The figure shows three views and two pictorial views of one solid part (mm, origin at its lowest corner). Answer the questions. A direction names the side the tool comes from. Round coordinates to 2 decimals unless told otherwise and drop trailing zeros. Write each loop counter-clockwise with the first axis right and the second up, starting at its lowest first coordinate (ties: lowest second). Pieces come first, ordered by that corner, then holes. Notation, with made-up numbers: M 66,64 L 121,64 A19 cw 121,91 Z; hole C 29.5,3.25 d6. An arc over 180 degrees is marked long. One line per item, written item: value. Start each with the question number.
Q1. Find section D-D (x = 4). Write down the section's boundary in (y, z).
Q2. The mould has two halves that part along X. Classify the marked faces 1, 2 and 3: released by +X, released by -X, zero draft, split by the parting line, or undercut.
Q3. Consider probe 1 along Y at (x, z) = (7.5, 1.25); probe 2 along Y at (x, z) = (7.5, 4.55); probe 3 along Z at (x, y) = (10.75, 4.5). Determine where each line is inside the solid, lowest interval first.
Q4. Given pin 1 Ø1 at (y, z) = (10, 3) entering from +X; pin 2 Ø2 at (y, z) = (13, 2) entering from -X; pin 3 Ø1.5 at (x, z) = (11.5, 5.5) entering from -Y, each flat-ended and moving along its own axis, determine where each tip first touches the part or whether it passes through.
Q5. A tool of negligible diameter and unlimited length cuts with its end or side. For the marked faces 4 and 5, from which of +Z, -Z, +X, -X, +Y, -Y can it reach the whole face along a straight path? Write none if from no direction.
Q6. Find section A-A (y = 7.5). Write down the section's boundary in (x, z), and give its area (3 significant figures).
Q7. Find section C-C (z = 1). Write down the section's boundary in (x, y).
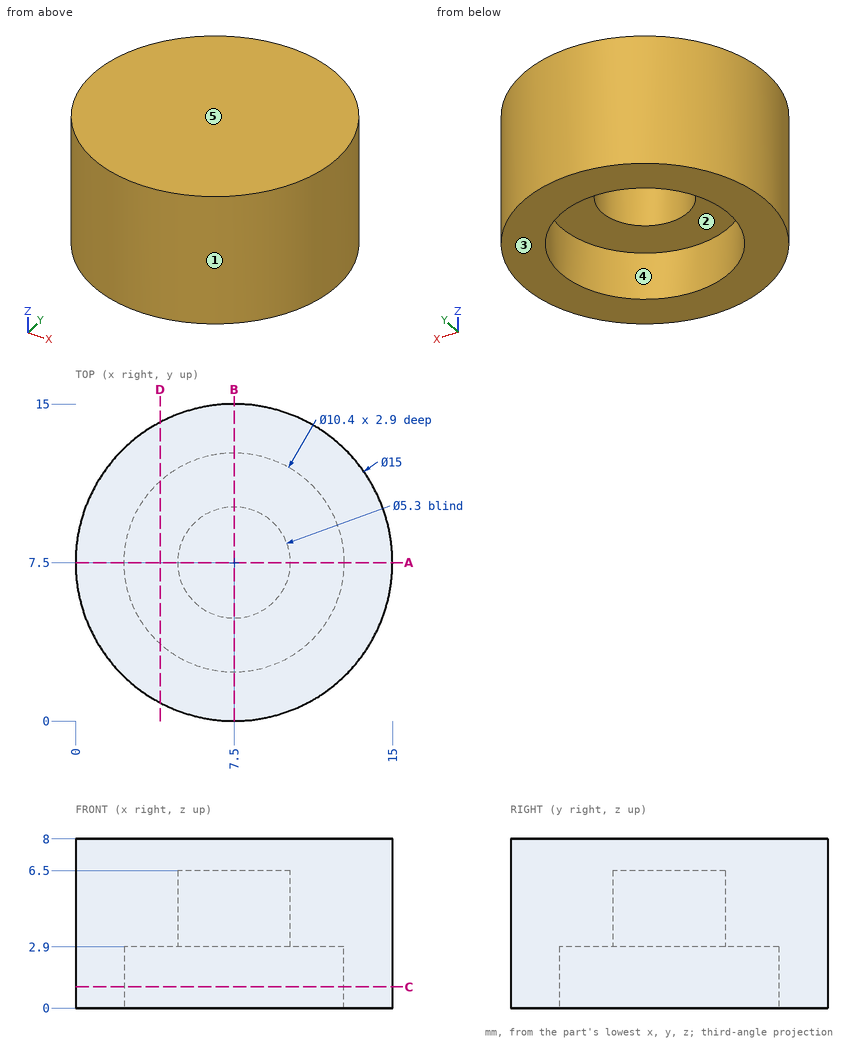
The answers:
1. outline: M 0.87,0 L 3.65,0 L 3.65,2.9 L 11.35,2.9 L 11.35,0 L 14.13,0 L 14.13,8 L 0.87,8 Z
2. face 1: split by the parting line
2. face 2: undercut
2. face 3: zero draft
3. probe 1: 0 to 2.3, 12.7 to 15
3. probe 2: 0 to 4.85, 10.15 to 15
3. probe 3: 2.9 to 8
4. pin 1: x = 14.73
4. pin 2: x = 1.5
4. pin 3: y = 0.74
5. face 4: -Z
5. face 5: +Z, +X, -X, +Y, -Y
6. outline: M 0,0 L 2.3,0 L 2.3,2.9 L 4.85,2.9 L 4.85,6.5 L 10.15,6.5 L 10.15,2.9 L 12.7,2.9 L 12.7,0 L 15,0 L 15,8 L 0,8 Z
6. area: 70.8 mm2
7. outline: C 7.5,7.5 d15; hole C 7.5,7.5 d10.4
